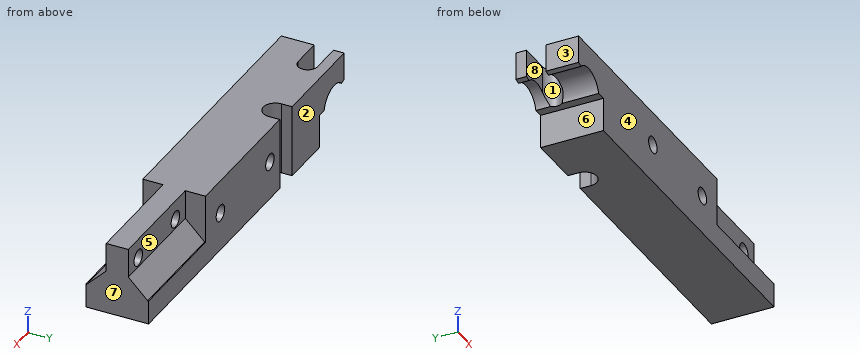
```python
from build123d import *

# Parameters (mm, degrees)
BOX001027045163_W      = 10
BOX001027045163_H      = 4
BOX001027045163_DEPTH  = 60
CYLINDER211_R          = 2
CYLINDER211_DEPTH      = 74
BOX001027045160_W      = 5
BOX001027045160_H      = 10
BOX001027045160_DEPTH  = 21
CYLINDER209_R          = 2.5
CYLINDER209_DEPTH      = 30
CYLINDER205_R          = 1.7
CYLINDER205_DEPTH      = 20
CYLINDER205_ROLL_ANGLE = 90
CYLINDER204_R          = 1.7
CYLINDER204_DEPTH      = 20
CYLINDER204_ROLL_ANGLE = 90
CYLINDER199_R          = 1.7
CYLINDER199_DEPTH      = 20
CYLINDER199_ROLL_ANGLE = 90
CYLINDER198_R          = 1.7
CYLINDER198_DEPTH      = 20
CYLINDER198_ROLL_ANGLE = 90
BOX001027045153_W      = 29
BOX001027045153_H      = 10
BOX001027045153_DEPTH  = 26
BOX001027045151_W      = 41
BOX001027045151_H      = 7
BOX001027045151_DEPTH  = 43
BOX001027045152_W      = 25
BOX001027045152_H      = 6
BOX001027045152_DEPTH  = 43
CYLINDER197_R          = 4.2
CYLINDER197_DEPTH      = 18
CYLINDER197_ROLL_ANGLE = 90
BOX001027045150_W      = 20
BOX001027045150_H      = 18
BOX001027045150_DEPTH  = 15
BOX001027045149_W      = 79
BOX001027045149_H      = 13
BOX001027045149_DEPTH  = 15
CHAMFER017_SIZE        = 2
CHAMFER026_SIZE        = 4
CHAMFER027_SIZE        = 4


with BuildPart() as cube211:
    # Box001027045163 → Box001027045163 (new body)
    with BuildSketch(Plane(origin=(-10, -2, -57), x_dir=(1, 0, 0), z_dir=(0, 0, 1))):
        with Locations((5, 2)):
            Rectangle(BOX001027045163_W, BOX001027045163_H)
    extrude(amount=BOX001027045163_DEPTH)


with BuildPart() as fusion112110:
    # Cylinder211 → Cylinder211 (new body)
    with BuildSketch(Plane.XY.offset(-62)):
        Circle(CYLINDER211_R)
    extrude(amount=CYLINDER211_DEPTH)

    # Fusion112110: union Cube211
    add(cube211.part)


with BuildPart() as fusion112110_1:
    # Fusion112110 placement: moved
    add(fusion112110.part.moved(Location((2.5, 0, 0))))


with BuildPart() as cube208:
    # Box001027045160 → Box001027045160 (new body)
    with BuildSketch(Plane(origin=(17, 2, -68), x_dir=(1, 0, 0), z_dir=(0, 0, 1))):
        with Locations((2.5, 5)):
            Rectangle(BOX001027045160_W, BOX001027045160_H)
    extrude(amount=BOX001027045160_DEPTH)


with BuildPart() as fusion112106:
    # Cylinder209 → Cylinder209 (new body)
    with BuildSketch(Plane(origin=(19.5, 2, -70), x_dir=(1, 0, 0), z_dir=(0, 0, 1))):
        Circle(CYLINDER209_R)
    extrude(amount=CYLINDER209_DEPTH)

    # Fusion112106: union Cube208
    add(cube208.part)


with BuildPart() as cylinder249:
    # Cylinder205 → Cylinder205 (new body)
    with BuildSketch(Plane.XY):
        Circle(CYLINDER205_R)
    extrude(amount=CYLINDER205_DEPTH)


with BuildPart() as cylinder249_1:
    # Cylinder205 roll: moved
    add(cylinder249.part.rotate(Axis((0, 0, 0), (1, 0, 0)), CYLINDER205_ROLL_ANGLE))


with BuildPart() as cylinder249_2:
    # Cylinder205 placement: moved
    add(cylinder249_1.part.moved(Location((46, 8, -54))))


with BuildPart() as fusion112103:
    # Cylinder204 → Cylinder204 (new body)
    with BuildSketch(Plane.XY):
        Circle(CYLINDER204_R)
    extrude(amount=CYLINDER204_DEPTH)


with BuildPart() as fusion112103_1:
    # Cylinder204 roll: moved
    add(fusion112103.part.rotate(Axis((0, 0, 0), (1, 0, 0)), CYLINDER204_ROLL_ANGLE))


with BuildPart() as fusion112103_2:
    # Cylinder204 placement: moved
    add(fusion112103_1.part.moved(Location((26, 8, -54))))

    # Fusion112103: union Cylinder249
    add(cylinder249_2.part)


with BuildPart() as fusion112103_3:
    # Fusion112103 placement: moved
    add(fusion112103_2.part.moved(Location((0, 0, -2))))


with BuildPart() as cylinder243:
    # Cylinder199 → Cylinder199 (new body)
    with BuildSketch(Plane.XY):
        Circle(CYLINDER199_R)
    extrude(amount=CYLINDER199_DEPTH)


with BuildPart() as cylinder243_1:
    # Cylinder199 roll: moved
    add(cylinder243.part.rotate(Axis((0, 0, 0), (1, 0, 0)), CYLINDER199_ROLL_ANGLE))


with BuildPart() as cylinder243_2:
    # Cylinder199 placement: moved
    add(cylinder243_1.part.moved(Location((71, 8, -54))))


with BuildPart() as fusion112100:
    # Cylinder198 → Cylinder198 (new body)
    with BuildSketch(Plane.XY):
        Circle(CYLINDER198_R)
    extrude(amount=CYLINDER198_DEPTH)


with BuildPart() as fusion112100_1:
    # Cylinder198 roll: moved
    add(fusion112100.part.rotate(Axis((0, 0, 0), (1, 0, 0)), CYLINDER198_ROLL_ANGLE))


with BuildPart() as fusion112100_2:
    # Cylinder198 placement: moved
    add(fusion112100_1.part.moved(Location((56, 8, -54))))

    # Fusion112100: union Cylinder243
    add(cylinder243_2.part)


with BuildPart() as fusion112100_3:
    # Fusion112100 placement: moved
    add(fusion112100_2.part.moved(Location((0, 0, 1))))


with BuildPart() as cube201:
    # Box001027045153 → Box001027045153 (new body)
    with BuildSketch(Plane(origin=(23, -2, -64), x_dir=(1, 0, 0), z_dir=(0, 0, 1))):
        with Locations((14.5, 5)):
            Rectangle(BOX001027045153_W, BOX001027045153_H)
    extrude(amount=BOX001027045153_DEPTH)


with BuildPart() as cut174:
    # Box001027045151 → Box001027045151 (new body)
    with BuildSketch(Plane(origin=(35, 0, -59), x_dir=(1, 0, 0), z_dir=(0, 0, 1))):
        with Locations((20.5, 3.5)):
            Rectangle(BOX001027045151_W, BOX001027045151_H)
    extrude(amount=BOX001027045151_DEPTH)

    # Cut174: cut Cube201
    add(cube201.part, mode=Mode.SUBTRACT)


with BuildPart() as fusion112099:
    # Box001027045152 → Box001027045152 (new body)
    with BuildSketch(Plane(origin=(52, -10.6, -59), x_dir=(1, 0, 0), z_dir=(0, 0, 1))):
        with Locations((12.5, 3)):
            Rectangle(BOX001027045152_W, BOX001027045152_H)
    extrude(amount=BOX001027045152_DEPTH)

    # Fusion112099: union Cut174
    add(cut174.part)


with BuildPart() as rocker_cut001:
    # Cylinder197 → Cylinder197 (new body)
    with BuildSketch(Plane.XY):
        Circle(CYLINDER197_R)
    extrude(amount=CYLINDER197_DEPTH)


with BuildPart() as rocker_cut001_1:
    # Cylinder197 roll: moved
    add(rocker_cut001.part.rotate(Axis((0, 0, 0), (1, 0, 0)), CYLINDER197_ROLL_ANGLE))


with BuildPart() as rocker_cut001_2:
    # Cylinder197 placement: moved
    add(rocker_cut001_1.part.moved(Location((0, 7, -58))))


with BuildPart() as fusion112098:
    # Box001027045150 → Box001027045150 (new body)
    with BuildSketch(Plane(origin=(-14, -11.8, -72), x_dir=(1, 0, 0), z_dir=(0, 0, 1))):
        with Locations((10, 9)):
            Rectangle(BOX001027045150_W, BOX001027045150_H)
    extrude(amount=BOX001027045150_DEPTH)

    # Fusion112098: union rocker-cut001
    add(rocker_cut001_2.part)


with BuildPart() as base_and_mount:
    # Box001027045149 → Box001027045149 (new body)
    with BuildSketch(Plane(origin=(-4, -8.8, -64), x_dir=(1, 0, 0), z_dir=(0, 0, 1))):
        with Locations((39.5, 6.5)):
            Rectangle(BOX001027045149_W, BOX001027045149_H)
    extrude(amount=BOX001027045149_DEPTH)

    # Cut173: cut Fusion112098
    add(fusion112098.part, mode=Mode.SUBTRACT)

    # Chamfer017
    chamfer017_edges = [base_and_mount.edges().sort_by_distance(p)[0] for p in [
        (-4, -2.3, -56.719375),
    ]]
    chamfer(chamfer017_edges, length=CHAMFER017_SIZE)

    # Cut175: cut Fusion112099
    add(fusion112099.part, mode=Mode.SUBTRACT)

    # Cut176: cut Fusion112100
    add(fusion112100_3.part, mode=Mode.SUBTRACT)

    # Cut179: cut Fusion112103
    add(fusion112103_3.part, mode=Mode.SUBTRACT)

    # Cut184: cut Fusion112106
    add(fusion112106.part, mode=Mode.SUBTRACT)

    # Cut189: cut Fusion112110
    add(fusion112110_1.part, mode=Mode.SUBTRACT)

    # Chamfer026
    chamfer026_edges = [base_and_mount.edges().sort_by_distance(p)[0] for p in [
        (63.5, 0, -59),
    ]]
    chamfer(chamfer026_edges, length=CHAMFER026_SIZE)

    # Chamfer027
    chamfer027_edges = [base_and_mount.edges().sort_by_distance(p)[0] for p in [
        (63.5, -4.6, -59),
    ]]
    chamfer(chamfer027_edges, length=CHAMFER027_SIZE)


solid = base_and_mount.part
```
The model under review builds one solid part; all positions refer to its coordinate system, in mm. Face numbers are marked on the shaded views. A direction names the side the tool comes from. Coordinates: 2 decimals unless noted, no trailing zeros. Write each loop counter-clockwise with the first axis right and the second up, starting at its lowest first coordinate (ties: lowest second). Pieces come first, ordered by that corner, then holes.
1) We need section A-A on z = -53. State the section outline as (x, y) points, then the cut area to 3 significant figures.
2) We need section D-D on x = 53. State the section outline as (y, z) points, then the cut area to 3 significant figures.
3) To check wall thickness, follow probe 1 along X at (y, z) = (-3.4, -53); probe 2 along X at (y, z) = (3, -62); probe 3 along X at (y, z) = (-1.4, -53). State the ranges of each line that lie inside material, in increasing order.
4) Clearance check with flat-ended pins moving along their axes: pin 1 Ø1 at (x, y) = (5, -3.5) entering from -Z; pin 2 Ø6.5 at (x, z) = (61.5, -52.5) entering from +Y; pin 3 Ø6 at (y, z) = (3, -57.5) entering from +X; pin 4 Ø1.1 at (y, z) = (3, -59) entering from -X. State where each tip first meets the part, or that it passes through.
5) We need section B-B on x = 26. State the section outline as (y, z) points, then the cut area to 3 significant figures.
6) Machinability: for the marked faces 5, 6, 7 and 8, which of the approach directions +Z, -Z, +X, -X, +Y, -Y give a long, thin tool a straight path to every point of the face, cutting with its end or side? Answer none if there is none.
7) We need section C-C on y = -6.5. State the section outline as (x, z) points.
8) The part is to be moulded in two halves that separate along Y. For the marked faces 1, 2, 3 and 4, say which applies: pulls with the +Y half, pulls with the -Y half, needs draft (parallel to the pull), parting line crosses it, or undercut.
Answer list:
1. outline: (-4, -8.8) - (52, -8.8) - (52, -4.6) - (54.3, -4.6) - (54.3, 0) - (52, 0) - (52, 4.2) - (22, 4.2) - (22, 2) arc R2.5 cw to (17, 2) - (17, 4.2) - (-4, 4.2) - (-4, 2) - (2.5, 2) arc R2 cw to (2.5, -2) - (-4, -2) - close; (57.7, -4.6) - (69.3, -4.6) - (69.3, 0) - (57.7, 0) - close; (72.7, -4.6) - (75, -4.6) - (75, 0) - (72.7, 0) - close
1. area: 749 mm2
2. outline: (-8.8, -64) - (4.2, -64) - (4.2, -59) - (4, -59) - (0, -55) - (0, -49) - (-4.6, -49) - (-4.6, -55) - (-8.6, -59) - (-8.8, -59) - close
2. area: 127 mm2
3. probe 1: x = -4 to 54.3, 57.7 to 69.3, 72.7 to 75
3. probe 2: x = 6 to 17, 22 to 75
3. probe 3: x = 3.93 to 54.3, 57.7 to 69.3, 72.7 to 75
4. pin 1: stops at z = -57
4. pin 2: stops at y = 0.75
4. pin 3: stops at x = 75
4. pin 4: stops at x = 6
5. outline: (-8.8, -64) - (4.2, -64) - (4.2, -57.7) - (-8.8, -57.7) - close; (-8.8, -54.3) - (4.2, -54.3) - (4.2, -49) - (-8.8, -49) - close
5. area: 151 mm2
6. face 5: +Z, +X, +Y
6. face 6: -Z, -X, +Y, -Y
6. face 7: +Z, -Z, +X, +Y, -Y
6. face 8: +Z, -Z, -X
7. outline: (-4, -54.72) - (-2.95, -55.01) arc R4.2 cw to (4.08, -57) - (6, -57) - (6, -64) - (75, -64) - (75, -56.9) - (52, -56.9) - (52, -49) - (-4, -49) - close; hole circle Ø3.4 at (26, -56); hole circle Ø3.4 at (46, -56)
8. face 1: undercut
8. face 2: pulls with the +Y half
8. face 3: needs draft
8. face 4: pulls with the -Y half
